```python
from build123d import *

# Parameters (mm, degrees)
BOSS_EXTRUDE1_DEPTH = 7.6
SKETCH2_5_W         = 85
SKETCH2_5_H         = 72
CUT_EXTRUDE9_DEPTH  = 1.61
CUT_EXTRUDE10_DEPTH = 2
SKETCH2_R           = 1.55
CUT_EXTRUDE3_DEPTH  = 90.547849587
FILLET1_R           = 5
SKETCH5_R           = 1.525
CUT_EXTRUDE4_DEPTH  = 10
SKETCH5_3_R         = 4.5
CUT_EXTRUDE5_DEPTH  = 1
CUT_EXTRUDE6_DEPTH  = 2.4
SKETCH12_R          = 2.75
SKETCH12_R_2        = 3
CUT_EXTRUDE11_DEPTH = 5
SKETCH2_6_W         = 86
SKETCH2_6_H         = 73
CUT_EXTRUDE12_DEPTH = 1.61


with BuildPart() as part:
    # Sketch1 → Boss-Extrude1 (new body)
    with BuildSketch(Plane(origin=(0, 0, 0), x_dir=(1, 0, 0), z_dir=(0, 1, 0))):
        Polygon((-40.307015775, 35.377886591), (-40.307015775, 7.377886591), (-55.307015775, 7.377886591), (-55.307015775, -17.622113409), (-44.307015775, -17.622113409), (45.692984225, -17.622113409), (65.692984225, -17.622113409), (65.692984225, 7.377886591), (50.692984225, 7.377886591), (50.692984225, 35.377886591), (65.692984225, 35.377886591), (65.692984225, 60.377886591), (45.692984225, 60.377886591), (-44.307015775, 60.377886591), (-55.307015775, 60.377886591), (-55.307015775, 35.377886591), align=None)
    extrude(amount=BOSS_EXTRUDE1_DEPTH)

    # Sketch2_5 → Cut-Extrude9 (cut)
    with BuildSketch(Plane(origin=(0, 7.6, 0), x_dir=(1, 0, 0), z_dir=(0, 1, 0))):
        with Locations((5.192984225, 21.377886591)):
            Rectangle(SKETCH2_5_W, SKETCH2_5_H)
    extrude(amount=-CUT_EXTRUDE9_DEPTH, mode=Mode.SUBTRACT)

    # Sketch11 → Cut-Extrude10 (cut)
    with BuildSketch(Plane(origin=(0, 5.99, 0), x_dir=(1, 0, 0), z_dir=(0, 1, 0))):
        Polygon((-35.999166331, 50.377886591), (-7.351072422, 50.377886591), (-7.351072422, 56.377886591), (3.851672568, 56.377886591), (3.851672568, 50.377886591), (47.692984225, 50.377886591), (47.692984225, 43.777886591), (39.692984225, 43.777886591), (39.692984225, 23.977886591), (47.692984225, 23.977886591), (47.692984225, 16.077886591), (44.692984225, 16.077886591), (44.692984225, -6.156199895), (38.382984225, -6.156199895), (38.382984225, -9.622113409), (7.110984225, -9.622113409), (7.110984225, -12.237769432), (3.110984225, -12.237769432), (3.110984225, -7.622113409), (-31.857233389, -7.622113409), (-31.857233389, -3.622113409), (-35.999166331, -3.622113409), (-35.999166331, 30.077886591), (-37.307015775, 30.077886591), (-37.307015775, 50.377886591), align=None)
    extrude(amount=-CUT_EXTRUDE10_DEPTH, mode=Mode.SUBTRACT)

    # Sketch2 → Cut-Extrude3 (cut, through all)
    with BuildSketch(Plane(origin=(0, 7.6, 0), x_dir=(1, 0, 0), z_dir=(0, 1, 0))):
        with Locations(Location((43.464984225, 53.313886591, 0), (0, 0, 270))):
            Circle(SKETCH2_R)
        with Locations(Location((-33.243015775, 53.313886591, 0), (0, 0, 270))):
            Circle(SKETCH2_R)
        with Locations(Location((-33.243015775, -10.558113409, 0), (0, 0, 270))):
            Circle(SKETCH2_R)
        with Locations(Location((43.464984225, -10.558113409, 0), (0, 0, 270))):
            Circle(SKETCH2_R)
    extrude(amount=-CUT_EXTRUDE3_DEPTH, mode=Mode.SUBTRACT)

    # Fillet1
    fillet1_edges = [part.edges().sort_by_distance(p)[0] for p in [
        (65.692984225, 3.8, -60.377886591),
        (65.692984225, 3.8, -35.377886591),
        (50.692984225, 3.8, -35.377886591),
        (50.692984225, 3.8, -7.377886591),
        (65.692984225, 3.8, -7.377886591),
        (65.692984225, 3.8, 17.622113409),
        (-55.307015775, 3.8, 17.622113409),
        (-55.307015775, 3.8, -7.377886591),
        (-40.307015775, 3.8, -7.377886591),
        (-40.307015775, 3.8, -35.377886591),
        (-55.307015775, 3.8, -35.377886591),
        (-55.307015775, 3.8, -60.377886591),
    ]]
    fillet(fillet1_edges, radius=FILLET1_R)

    # Sketch5 → Cut-Extrude4 (cut)
    with BuildSketch(Plane(origin=(0, 7.6, 0), x_dir=(1, 0, 0), z_dir=(0, 1, 0))):
        with Locations(Location((-47.807015775, 52.877886591, 0), (0, 0, 270))):
            Circle(SKETCH5_R)
        with Locations(Location((-47.807015775, -10.122113409, 0), (0, 0, 270))):
            Circle(SKETCH5_R)
        with Locations(Location((58.192984225, -10.122113409, 0), (0, 0, 270))):
            Circle(SKETCH5_R)
        with Locations(Location((58.192984225, 52.877886591, 0), (0, 0, 270))):
            Circle(SKETCH5_R)
        with Locations(Location((-47.807015775, 40.377886591, 0), (0, 0, 270))):
            Circle(SKETCH5_R)
        with Locations(Location((-47.807015775, 2.377886591, 0), (0, 0, 270))):
            Circle(SKETCH5_R)
        with Locations(Location((58.192984225, 2.377886591, 0), (0, 0, 270))):
            Circle(SKETCH5_R)
        with Locations(Location((58.192984225, 40.377886591, 0), (0, 0, 270))):
            Circle(SKETCH5_R)
    extrude(amount=-CUT_EXTRUDE4_DEPTH, mode=Mode.SUBTRACT)

    # Sketch5_3 → Cut-Extrude5 (cut)
    with BuildSketch(Plane(origin=(0, 7.6, 0), x_dir=(1, 0, 0), z_dir=(0, 1, 0))):
        with Locations(Location((-47.807015775, 52.877886591, 0), (0, 0, 270))):
            Circle(SKETCH5_3_R)
    extrude(amount=-CUT_EXTRUDE5_DEPTH, mode=Mode.SUBTRACT)

    # Sketch6 → Cut-Extrude6 (cut)
    with BuildSketch(Plane.XZ):
        Polygon((-48.06313711, 6.92807179), (-45.16895526, 8.303285016), (-44.912833924, 11.497326635), (-47.550894439, 13.316155027), (-50.445076289, 11.940941801), (-50.701197625, 8.746900183), align=None)
        Polygon((57.994664168, 6.923962513), (60.863504118, 8.351287753), (61.061824175, 11.549438649), (58.391304282, 13.320264305), (55.522464333, 11.892939064), (55.324144276, 8.694788168), align=None)
        Polygon((60.566668821, -50.725417907), (57.515733962, -49.745981088), (55.142049366, -51.898449773), (55.819299629, -55.030355276), (58.870234489, -56.009792094), (61.243919085, -53.85732341), align=None)
        Polygon((-51.011308362, -52.874883962), (-49.411762421, -55.651384058), (-46.207469834, -55.654386687), (-44.602723187, -52.88088922), (-46.202269128, -50.104389124), (-49.406561715, -50.101386495), align=None)
        Polygon((-36.168627764, 11.865130811), (-35.837732042, 8.677967805), (-32.912120053, 7.370950404), (-30.317403786, 9.251096007), (-30.648299507, 12.438259012), (-33.573911496, 13.745276414), align=None)
        Polygon((40.267307985, 10.763945049), (41.687890676, 7.891760372), (44.885566916, 7.685928731), (46.662660465, 10.352281768), (45.242077775, 13.224466445), (42.044401535, 13.430298086), align=None)
        Polygon((40.985735994, -55.343868908), (43.983376365, -56.4759697), (46.462624597, -54.445987383), (45.944232457, -51.283904274), (42.946592085, -50.151803482), (40.467343854, -52.181785799), align=None)
        Polygon((-36.426218549, -53.680928955), (-34.51674915, -56.254142241), (-31.333546376, -55.887099877), (-30.059813, -52.946844227), (-31.969282399, -50.373630941), (-35.152485173, -50.740673305), align=None)
    extrude(amount=-CUT_EXTRUDE6_DEPTH, mode=Mode.SUBTRACT)

    # Sketch12 → Cut-Extrude11 (cut)
    with BuildSketch(Plane(origin=(0, 5.99, 0), x_dir=(1, 0, 0), z_dir=(0, 1, 0))):
        with Locations(Location((28.732984225, 19.667886591, 0), (0, 0, 270))):
            Circle(SKETCH12_R)
        with Locations(Location((44.992984225, 19.667886591, 0), (0, 0, 270))):
            Circle(SKETCH12_R)
        with Locations(Location((-17.305374837, 3.407886591, 0), (0, 0, 270))):
            Circle(SKETCH12_R_2)
        with Locations(Location((-17.305374837, 23.477886591, 0), (0, 0, 270))):
            Circle(SKETCH12_R_2)
    extrude(amount=-CUT_EXTRUDE11_DEPTH, mode=Mode.SUBTRACT)

    # Sketch2_6 → Cut-Extrude12 (cut)
    with BuildSketch(Plane(origin=(0, 7.6, 0), x_dir=(1, 0, 0), z_dir=(0, 1, 0))):
        with Locations((5.192984225, 21.377886591)):
            Rectangle(SKETCH2_6_W, SKETCH2_6_H)
    extrude(amount=-CUT_EXTRUDE12_DEPTH, mode=Mode.SUBTRACT)


solid = part.part
```
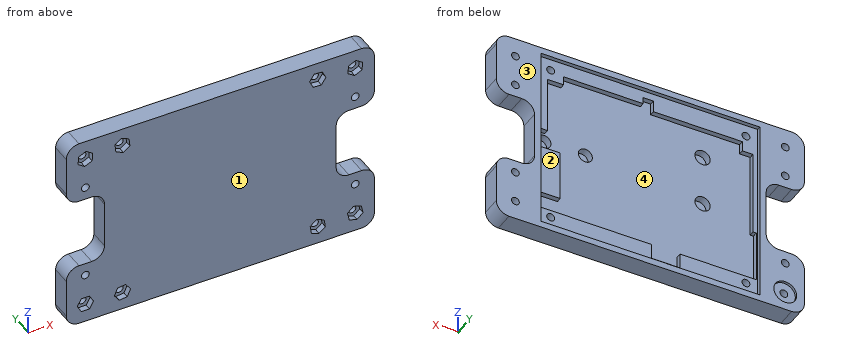
Geometry: final body of the model. Coordinates: model frame, mm. Face numbers are marked on the shaded views. A direction names the side the tool comes from. Coordinates: 2 decimals unless noted, no trailing zeros. Loops run counter-clockwise (first coordinate to the right, second up) from the corner with the lowest first, then second, coordinate; pieces in that order, holes last. Notation, with made-up numbers: (-19, 3.25) -> (0, 3.25) arc R12 ccw to (0, 24.25) -> close; hole circle Ø1 at (51.25, 19.5). An arc over 180 degrees is marked (long way). Use a Markdown table: item, result. Add a question column.
(1) Pin query (flat end, axial travel): pin 1 Ø1 at (y, z) = (3.5, -12) entering from -X; pin 2 Ø4 at (x, z) = (-19, -19) entering from +Y; pin 3 Ø3 at (x, z) = (-17, -23.5) entering from +Y. Return the tip coordinate at first contact, or that it passes through.
(2) Access query for the marked faces 1 and 2. Directions: +Z, -Z, +X, -X, +Y, -Y. A direction counts if a zero-diameter tool reaches every point of the face in a straight line with its end or side. Return the directions, or none.
(3) Section query C-C, the plane x = 9. Return loops of the section in (y, z), plus the area to 3 significant figures.
(4) Section query B-B, the plane x = -41.5. Return loops of the section in (y, z).
(5) Line query: line 1 along X through (y, z) = (6.75, -53); line 2 along X through (y, z) = (3.25, -20); line 3 along X through (y, z) = (5.25, -51). Output: solid intervals per line, ascending.
(6) Mould query, pull axis Z, two halves, no side actions, for the marked faces 3 and 4. Classes: pulls with the +Z half, pulls with the -Z half, needs draft (parallel to the pull), parting line crosses it, or undercut.
(7) Section query A-A, the plane z = -47. Return loops of the section in (x, y), plus the area to 3 significant figures.
Answer:
| question | item | result |
|---|---|---|
| 1 | pin 1 | stops at x = -40.38 |
| 1 | pin 2 | stops at y = 3.99 |
| 1 | pin 3 | stops at y = 0.99 |
| 2 | face 1 | +Z, -Z, +X, -X, -Y |
| 2 | face 2 | +Y |
| 3 | outline | (0, -60.38) -> (7.6, -60.38) -> (7.6, -57.88) -> (5.99, -57.88) -> (5.99, -50.38) -> (3.99, -50.38) -> (3.99, 9.62) -> (5.99, 9.62) -> (5.99, 15.12) -> (7.6, 15.12) -> (7.6, 17.62) -> (0, 17.62) -> close |
| 3 | area | 355 mm^2 |
| 4 | outline | (0, -60.38) -> (7.6, -60.38) -> (7.6, -33.62) -> (0, -33.62) -> close; (0, -9.14) -> (7.6, -9.14) -> (7.6, 17.62) -> (0, 17.62) -> close |
| 5 | line 1 | x = -55.31 to -52.31, -43.31 to -37.81, 48.19 to 56.67, 59.71 to 65.69 |
| 5 | line 2 | x = -40.31 to 26, 31.46 to 42.26, 47.72 to 50.69 |
| 5 | line 3 | x = -55.31 to -7.35, 3.85 to 65.69 |
| 6 | face 3 | needs draft |
| 6 | face 4 | undercut |
| 7 | outline | (-55.31, 0) -> (65.69, 0) -> (65.69, 7.6) -> (48.19, 7.6) -> (48.19, 5.99) -> (47.69, 5.99) -> (47.69, 3.99) -> (-37.31, 3.99) -> (-37.31, 5.99) -> (-37.81, 5.99) -> (-37.81, 7.6) -> (-55.31, 7.6) -> close |
| 7 | area | 611 mm^2 |
